from build123d import *

# Parameters (mm, degrees)
SKETCH2_W           = 29.3
SKETCH2_H           = 14.7
BOSS_EXTRUDE1_DEPTH = 22.9
BOSS_EXTRUDE2_START = 5
BOSS_EXTRUDE2_DEPTH = 6.35
SKETCH8_R           = 1
CUT_EXTRUDE3_DEPTH  = 0.9
SKETCH5_R           = 2
CUT_EXTRUDE1_DEPTH  = 3.2
CIRPATTERN1_COUNT   = 26
SKETCH7_W           = 0.55
SKETCH7_H           = 4
CUT_EXTRUDE2_DEPTH  = 17.523822727
FILLET1_R           = 0.1
FILLET1_2_R         = 1


with BuildPart() as part:
    # Sketch2 → Boss-Extrude1 (new body)
    with BuildSketch(Plane(origin=(0, 0, 0), x_dir=(1, 0, 0), z_dir=(0, 1, 0))):
        Rectangle(SKETCH2_W, SKETCH2_H)
    extrude(amount=BOSS_EXTRUDE1_DEPTH)

    # Sketch3 → Revolve1 (revolve)
    with BuildSketch(Plane.XY):
        Polygon((0, 22.9), (0, 33.9), (-3.72, 33.9), (-4.35, 33.27), (-4.35, 32.3), (-4.95, 32.3), (-5.35, 31.9), (-5.35, 31.6), (-9.21, 31.6), (-9.21, 28.4), (-5.35, 28.4), (-5.35, 24.4), (-6, 24.4), (-6, 22.9), align=None)
    revolve(axis=Axis((0, 22.9, 0), (0, 1, 0)))

    # Sketch4 → Boss-Extrude2 (add)
    with BuildSketch(Plane(origin=(0, 0, 0), x_dir=(0, 0, -1), z_dir=(1, 0, 0)).offset(BOSS_EXTRUDE2_START)):
        Polygon((-0.45, -4), (0.45, -4), (7.55, -4), (7.55, -3.1), (0.45, -3.1), (0.45, 0), (-0.45, 0), align=None)
    boss_extrude2 = extrude(amount=BOSS_EXTRUDE2_DEPTH)

    # Sketch8 → Cut-Extrude3 (cut)
    with BuildSketch(Plane.XZ.offset(4)):
        with Locations((8.175, -5.55)):
            Circle(SKETCH8_R)
    cut_extrude3 = extrude(amount=-CUT_EXTRUDE3_DEPTH, mode=Mode.SUBTRACT)

    # Mirror1: Boss-Extrude2, Cut-Extrude3 across plane
    add(boss_extrude2.mirror(Plane(origin=(0, 0, 0), x_dir=(0, 0, 1), z_dir=(1, 0, 0))))
    add(cut_extrude3.mirror(Plane(origin=(0, 0, 0), x_dir=(0, 0, 1), z_dir=(1, 0, 0))), mode=Mode.SUBTRACT)

    # Sketch5 → Cut-Extrude1 (cut)
    with BuildSketch(Plane(origin=(0, 31.6, 0), x_dir=(1, 0, 0), z_dir=(0, 1, 0))):
        with Locations((0, 11)):
            Circle(SKETCH5_R)
    cut_extrude1 = extrude(amount=-CUT_EXTRUDE1_DEPTH, mode=Mode.SUBTRACT)

    # CirPattern1: Cut-Extrude1 ×26 about axis
    cirpattern1_axis = Axis((0, 0, 0), (0, 1, 0))
    for i in range(1, CIRPATTERN1_COUNT):
        add(cut_extrude1.rotate(cirpattern1_axis, i * 360 / CIRPATTERN1_COUNT), mode=Mode.SUBTRACT)

    # Sketch7 → Cut-Extrude2 (cut, through all)
    with BuildSketch(Plane.XY.offset(7.35)):
        with Locations((5.075, 26.4)):
            Rectangle(SKETCH7_W, SKETCH7_H)
        with Locations((-5.075, 26.4)):
            Rectangle(SKETCH7_W, SKETCH7_H)
    extrude(amount=-CUT_EXTRUDE2_DEPTH, mode=Mode.SUBTRACT)

    # Fillet1
    fillet1_edges = [part.edges().sort_by_distance(p)[0] for p in [
        (8.175, -3.1, -0.45),
        (-8.175, -3.1, -0.45),
    ]]
    fillet(fillet1_edges, radius=FILLET1_R)

    # Fillet1 2
    fillet1_2_edges = [part.edges().sort_by_distance(p)[0] for p in [
        (8.175, -4, 0.45),
        (-8.175, -4, 0.45),
    ]]
    fillet(fillet1_2_edges, radius=FILLET1_2_R)


solid = part.part
Work out the finished part from the listing and answer in its coordinate system (mm). A direction names the side the tool comes from. Give positions to 0.01 mm unless a question says otherwise; leave off trailing zeros. Order: outer loops, then holes, each group sorted by start corner. A loop starts at its lowest first (then second) coordinate and runs counter-clockwise, first axis right, second up. Notation, with made-up numbers: M -2,-37 L 19,-37 A10 cw 19,-31 Z; hole C 54.5,69 d6. An arc over 180 degrees is marked long. Return JSON: item names as keys, results as strings.
Q1. Each of these flat-tipped pins is pushed along its axis until it touches: pin 1 (1 mm diameter, centred on x = -8.5, z = 4.5, fed in from +Y); pin 2 (1.5 mm diameter, centred on x = 5, y = 27.5, fed in from +Z); pin 3 (1.2 mm diameter, centred on x = -8.175, z = -5.55, fed in from -Y); pin 4 (2 mm diameter, centred on y = -2, z = -3, fed in from +X). Where does it stop, or does it pass through?
Answer below:
{"pin 1": "stops at y = 31.6", "pin 2": "stops at z = 3.25", "pin 3": "stops at y = 0", "pin 4": "passes through"}
Q2. The mould has two halves that part along Y. Classify faces 4 (the face through (-8, -1, 0.45)), 5 (the face through (8, -2, -0.45)), 6 (the face through (8, -4, -4)): pulls with the +Y half, pulls with the -Y half, needs draft (parallel to the pull), parting line crosses it, or undercut.
Answer below:
{"face 4": "needs draft", "face 5": "undercut", "face 6": "pulls with the -Y half"}
Q3. Find section A-A, the plane y = -2. Write down the section's boundary in (x, z), and give its area (3 significant figures).
Answer below:
{"outline": "M -11.35,-0.45 L -5,-0.45 L -5,0.45 L -11.35,0.45 Z; M 5,-0.45 L 11.35,-0.45 L 11.35,0.45 L 5,0.45 Z", "area": "11.4 mm^2"}
Q4. Find section B-B, the plane y = 14. Write down the section's boundary in (x, z), and give its area (3 significant figures).
Answer below:
{"outline": "M -14.65,-7.35 L 14.65,-7.35 L 14.65,7.35 L -14.65,7.35 Z", "area": "431 mm^2"}
Q5. Which of the six approach directions +Z, -Z, +X, -X, +Y, -Y give full straight-line access (tool end or side, diameter ignored) to faces 1 (the face through (5.977, 30.022, 6.729)), 2 (the face through (-8.933, 30.022, 1.097)), 3 (the face through (7.4, 30.02, -5.12))?
Answer below:
{"face 1": "+Z, +X, +Y", "face 2": "-X, +Y", "face 3": "-Z, +X, +Y"}
Q6. Find the intervals of material crossed by line 1 along Y through (x, z) = (7.5, 1.5); line 2 along Z through (x, y) = (-9, 17.5); line 3 along Y through (x, z) = (13, 3.5), in increasing order. Write a range as [from, to].
Answer below:
{"line 1": "y = [0, 22.9], [28.4, 31.6]", "line 2": "z = [-7.35, 7.35]", "line 3": "y = [0, 22.9]"}
